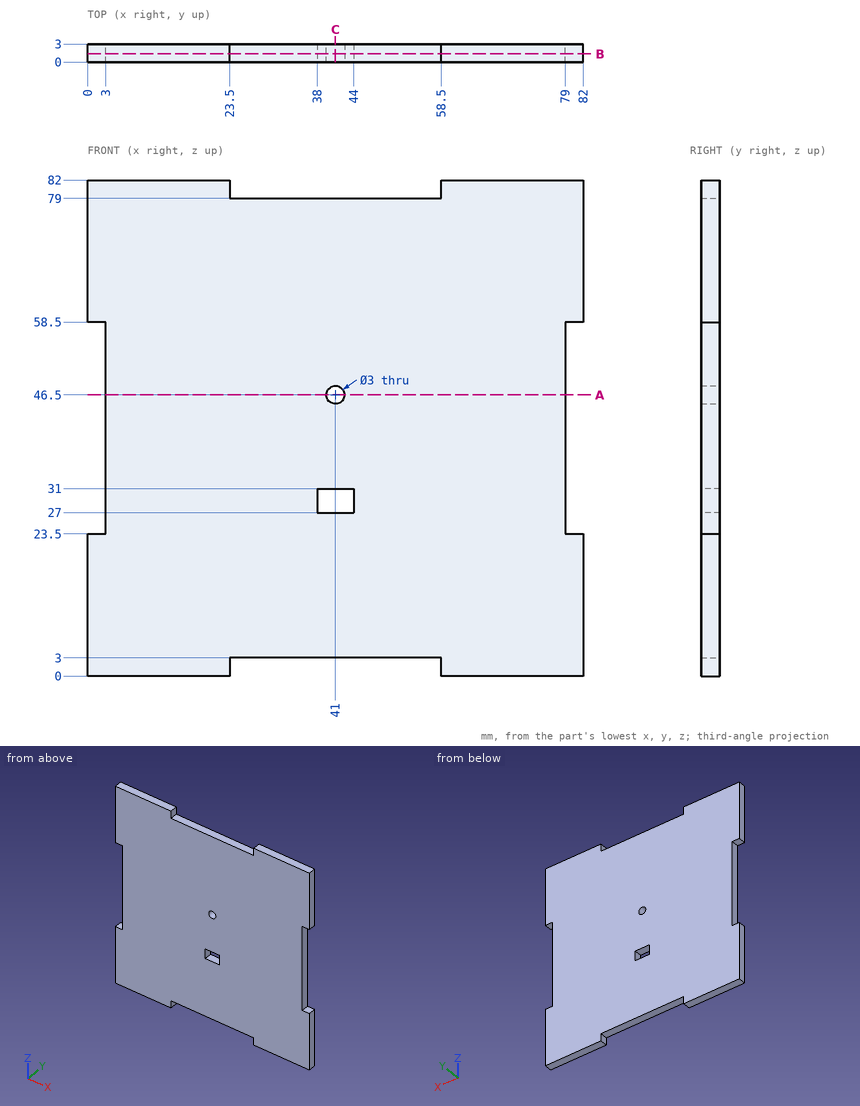
Part print with two shaded views. Sizes in mm from the minimum x, y, z corner. Coordinates: 2 decimals unless noted, no trailing zeros. Order: outer loops, then holes, each group sorted by start corner. A loop starts at its lowest first (then second) coordinate and runs counter-clockwise, first axis right, second up. Notation, with made-up numbers: (41.5, 30) - (86.5, 30) arc R19 ccw to (86.5, 47) - close; hole circle Ø7 at (3.25, 87). An arc over 180 degrees is marked (long way). Answer in a Markdown table with one row per item.
1. Slice it at C-C, the plane x = 41. List the corners of the cut face in (y, z).
Answer:
| item | result |
|---|---|
| outline | (0, 3) - (3, 3) - (3, 27) - (0, 27) - close; (0, 31) - (3, 31) - (3, 45) - (0, 45) - close; (0, 48) - (3, 48) - (3, 79) - (0, 79) - close |
2. Slice it at B-B, the plane y = 1.35. List the corners of the cut face in (x, z), then the cut area to 3 significant figures.
Answer:
| item | result |
|---|---|
| outline | (0, 0) - (23.5, 0) - (23.5, 3) - (58.5, 3) - (58.5, 0) - (82, 0) - (82, 23.5) - (79, 23.5) - (79, 58.5) - (82, 58.5) - (82, 82) - (58.5, 82) - (58.5, 79) - (23.5, 79) - (23.5, 82) - (0, 82) - (0, 58.5) - (3, 58.5) - (3, 23.5) - (0, 23.5) - close; hole (38, 27) - (44, 27) - (44, 31) - (38, 31) - close; hole circle Ø3 at (41, 46.5) |
| area | 6,270 mm² |
3. Slice it at A-A, the plane z = 46.5. List the corners of the cut face in (x, y), then the cut area to 3 significant figures.
Answer:
| item | result |
|---|---|
| outline | (3, 0) - (39.5, 0) - (39.5, 3) - (3, 3) - close; (42.5, 0) - (79, 0) - (79, 3) - (42.5, 3) - close |
| area | 219 mm² |
4. Flat gauge pins, fed straight in: P1, Ø10, axis at x = 28, z = 25.5, coming from the -Y side; P2, Ø1.5, axis at x = 40.5, y = 1, coming from the +Z side; P3, Ø0.9, axis at x = 42, y = 1.5, coming from the -Z side; P4, Ø1.5, axis at y = 2, z = 35.5, coming from the -X side. Where does each tip first touch, or does it go through?
Answer:
| item | result |
|---|---|
| P1 | y = 0 |
| P2 | z = 79 |
| P3 | z = 3 |
| P4 | x = 3 |
5. Drill centre lines: L1, parallel to Z at x = 41, y = 1.95; L2, parallel to X at y = 0.85, z = 46.5; L3, parallel to Z at x = 54.5, y = 1.85. Where is each one in solid material? Low to high. Write a range as from..to.
Answer:
| item | result |
|---|---|
| L1 | 3..27, 31..45, 48..79 |
| L2 | 3..39.5, 42.5..79 |
| L3 | 3..79 |
